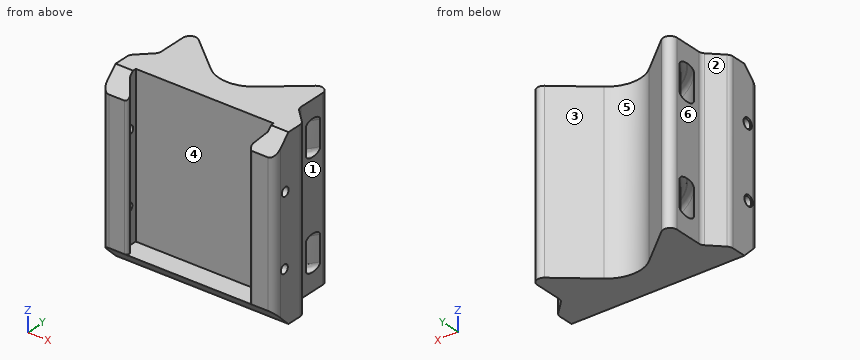
from build123d import *

# Parameters (mm, degrees)
BOSS_EXTRUDE1_DEPTH             = 50
SKETCH2_W                       = 10
SKETCH2_H                       = 3
M3X0_5_TAPPED_HOLE1_D           = 2.5
M3X0_5_TAPPED_HOLE1_CSINK_D     = 3.05
M3X0_5_TAPPED_HOLE1_CSINK_ANGLE = 90
FILLET2_R                       = 1.4
SKETCH5_W                       = 42.664543816
SKETCH5_H                       = 6
BOSS_EXTRUDE2_DEPTH             = 5
CUT_EXTRUDE1_DEPTH              = 70.875165408
CUT_EXTRUDE1_DEPTH_BACK         = 70.875165408


with BuildPart() as part:
    # Sketch1 → Boss-Extrude1 (new body)
    with BuildSketch(Plane.XY):
        with BuildLine():
            Line((6.427876097, 10.393628462), (16.714424781, 19.025067669))
            ThreePointArc((16.714424781, 19.025067669), (18.845236523, 19.305594357), (20, 17.492978783))
            Line((20, 17.492978783), (20, 9.578427125))
            ThreePointArc((20, 9.578427125), (20.152240935, 8.81306026), (20.585786438, 8.164213562))
            Line((20.585786438, 8.164213562), (24.164213562, 4.585786438))
            ThreePointArc((24.164213562, 4.585786438), (24.597759065, 3.93693974), (24.75, 3.171572875))
            Line((24.75, 3.171572875), (24.75, -4))
            ThreePointArc((24.75, -4), (24.164213562, -5.414213562), (22.75, -6))
            Line((22.75, -6), (18.277026938, -6))
            ThreePointArc((18.277026938, -6), (17.551980708, -5.538094609), (17.664191383, -4.685769912))
            Line((17.664191383, -4.685769912), (19.75, -2.2))
            Line((19.75, -2.2), (19.75, 0))
            Line((19.75, 0), (-19.75, 0))
            Line((-19.75, 0), (-19.75, -2.2))
            Line((-19.75, -2.2), (-17.664191383, -4.685769912))
            ThreePointArc((-17.664191383, -4.685769912), (-17.551980708, -5.538094609), (-18.277026938, -6))
            Line((-18.277026938, -6), (-22.75, -6))
            ThreePointArc((-22.75, -6), (-24.164213562, -5.414213562), (-24.75, -4))
            Line((-24.75, -4), (-24.75, 3.171572875))
            ThreePointArc((-24.75, 3.171572875), (-24.597759065, 3.93693974), (-24.164213562, 4.585786438))
            Line((-24.164213562, 4.585786438), (-20.585786438, 8.164213562))
            ThreePointArc((-20.585786438, 8.164213562), (-20.152240935, 8.81306026), (-20, 9.578427125))
            Line((-20, 9.578427125), (-20, 17.492978783))
            ThreePointArc((-20, 17.492978783), (-18.845236523, 19.305594357), (-16.714424781, 19.025067669))
            Line((-16.714424781, 19.025067669), (-6.427876097, 10.393628462))
            ThreePointArc((-6.427876097, 10.393628462), (0, 8.054072893), (6.427876097, 10.393628462))
        make_face()
    extrude(amount=BOSS_EXTRUDE1_DEPTH)

    # Sketch2 → Cut-Revolve1 (revolve, cut)
    with BuildSketch(Plane(origin=(0, 0, 0), x_dir=(0, 0, -1), z_dir=(1, 0, 0))):
        with Locations((-10, 3.5)):
            Rectangle(SKETCH2_W, SKETCH2_H)
        with Locations((-40, 3.5)):
            Rectangle(SKETCH2_W, SKETCH2_H)
    revolve(axis=Axis((0, 28.054072893, 39.353848425), (0, 0, -1)), mode=Mode.SUBTRACT)

    # M3x0.5 Tapped Hole1 (through all)
    with Locations(Plane.ZY.offset(24.75)):
        with Locations((15, -2.5), (34.997686823, -2.195826159)):
            CounterSinkHole(M3X0_5_TAPPED_HOLE1_D / 2, M3X0_5_TAPPED_HOLE1_CSINK_D / 2, counter_sink_angle=M3X0_5_TAPPED_HOLE1_CSINK_ANGLE)

    # Fillet2
    fillet2_edges = [part.edges().sort_by_distance(p)[0] for p in [
        (0, 5, 5),
        (0, 2, 5),
        (0, 2, 15),
        (0, 5, 15),
        (0, 5, 35),
        (0, 2, 35),
        (0, 2, 45),
        (0, 5, 45),
    ]]
    fillet(fillet2_edges, radius=FILLET2_R)

    # Sketch5 → Boss-Extrude2 (add)
    with BuildSketch(Plane(origin=(0, 0, 0), x_dir=(-1, 0, 0), z_dir=(0, 0, -1))):
        with Locations((-0.389940088, -3)):
            Rectangle(SKETCH5_W, SKETCH5_H)
    extrude(amount=-BOSS_EXTRUDE2_DEPTH)

    # Sketch6 → Cut-Extrude1 (cut, two sides: drawn at the far end of the back side and taken through both)
    with BuildSketch(Plane(origin=(20, 0, 0), x_dir=(0, 0, -1), z_dir=(1, 0, 0)).offset(-CUT_EXTRUDE1_DEPTH_BACK)):
        Polygon((-50, 32.923814778), (-50, -1), (-45, -6), (-5, -6), (0, -1), (0, 27.637517517), (9.715724937, 27.637517517), (9.715724937, -14.512697257), (-61.049340823, -14.512697257), (-61.049340823, 32.923814778), align=None)
    extrude(amount=CUT_EXTRUDE1_DEPTH + CUT_EXTRUDE1_DEPTH_BACK, mode=Mode.SUBTRACT)


solid = part.part
Could you check a few things on this model? Use its own coordinates, in mm. Face numbers are marked on the shaded views. A direction names the side the tool comes from. Give positions to 0.01 mm unless a question says otherwise; leave off trailing zeros. Write each loop counter-clockwise with the first axis right and the second up, starting at its lowest first coordinate (ties: lowest second). Pieces come first, ordered by that corner, then holes. Notation, with made-up numbers: (-30, -23.5) - (16, -23.5) arc R13 ccw to (16, -0.5) - close; hole circle Ø8 at (45, -8.5). An arc over 180 degrees is marked (long way). Use CSV: the item, a comma, the result in double quotes. Start each with the question number.
Item 1: I want a section at B-B, the plane z = 28.5. Please give me the cut outline in (x, y), then the cut area to 3 significant figures.
Item 2: If I drill on line 1 along X through (y, z) = (-0.5, 29); line 2 along Z through (x, y) = (19.5, -1); line 3 along Z through (x, y) = (-22.5, -2.5), over which ranges is the centre line in solid material (lowest first)?
Item 3: If we mould it in two halves opening along X, with no side actions, what happens to the marked faces 1, 2, 3 and 4? For each: pulls with the +X half, pulls with the -X half, needs draft (parallel to the pull), parting line crosses it, or undercut.
Item 4: I'm going to push flat-ended pins straight in: pin 1 (5 mm diameter, centred on x = 9, y = -3, fed in from +Z); pin 2 (3 mm diameter, centred on y = -2.5, z = 15, fed in from -X) (3 decimals); pin 3 (4 mm diameter, centred on y = 13.5, z = 32.5, fed in from -X). Where does each tip first touch, or does it pass through?
Item 5: I want a section at A-A, the plane x = 0. Please give me the cut outline in (y, z).
Item 6: For the marked faces 5 and 6, which set-ups out of +Z, -Z, +X, -X, +Y, -Y let a thin tool reach every point of the face, with its end or its side?
Item 7: I want a section at C-C, the plane y = 6.75. Give the number of separate pieces and of enclosed holes in the cut face, then the cut area to 3 significant figures.
Findings:
1,outline,"(-24.75, -4) arc R2 ccw to (-22.75, -6) - (-18.28, -6) arc R0.8 ccw to (-17.66, -4.69) - (-19.75, -2.2) - (-19.75, 0) - (19.75, 0) - (19.75, -2.2) - (17.66, -4.69) arc R0.8 ccw to (18.28, -6) - (22.75, -6) arc R2 ccw to (24.75, -4) - (24.75, 3.17) arc R2 ccw to (24.16, 4.59) - (20.59, 8.16) arc R2 cw to (20, 9.58) - (20, 17.49) arc R2 ccw to (16.71, 19.03) - (6.43, 10.39) arc R10 cw to (-6.43, 10.39) - (-16.71, 19.03) arc R2 ccw to (-20, 17.49) - (-20, 9.58) arc R2 cw to (-20.59, 8.16) - (-24.16, 4.59) arc R2 ccw to (-24.75, 3.17) - close"
1,area,"671 mm2"
2,line 1,"x = -24.75 to -19.75, 19.75 to 24.75"
2,line 2,"z = 0 to 5"
2,line 3,"z = 1.5 to 13.75, 16.25 to 33.79, 36.21 to 48.5"
3,face 1,"pulls with the +X half"
3,face 2,"pulls with the -X half"
3,face 3,"undercut"
3,face 4,"undercut"
4,pin 1,"stops at z = 5"
4,pin 2,"stops at x = -24.725"
4,pin 3,"stops at x = -20"
5,outline,"(-6, 5) - (-1, 0) - (8.05, 0) - (8.05, 50) - (0, 50) - (0, 5) - close; hole (2, 6.4) arc R1.4 ccw to (3.4, 5) - (3.6, 5) arc R1.4 ccw to (5, 6.4) - (5, 13.6) arc R1.4 ccw to (3.6, 15) - (3.4, 15) arc R1.4 ccw to (2, 13.6) - close; hole (2, 36.4) arc R1.4 ccw to (3.4, 35) - (3.6, 35) arc R1.4 ccw to (5, 36.4) - (5, 43.6) arc R1.4 ccw to (3.6, 45) - (3.4, 45) arc R1.4 ccw to (2, 43.6) - close"
6,face 5,"+Z, -Z, +Y"
6,face 6,"+Z, -Z, -X, +Y"
7,separate pieces,"1"
7,enclosed holes,"4"
7,area,"1,970 mm2"
